Design review of the part shown in the three views and the two pictorial views. Dimensions are in mm from the part's minimum x, y and z. Give positions to 0.01 mm unless a question says otherwise; leave off trailing zeros. Order: outer loops, then holes, each group sorted by start corner. A loop starts at its lowest first (then second) coordinate and runs counter-clockwise, first axis right, second up. Notation, with made-up numbers: (-10, -30.75) - (29, -30.75) arc R29 cw to (29, -10.75) - close; hole circle Ø3 at (11.25, 6). An arc over 180 degrees is marked (long way). Put each result on its own line as item: value.
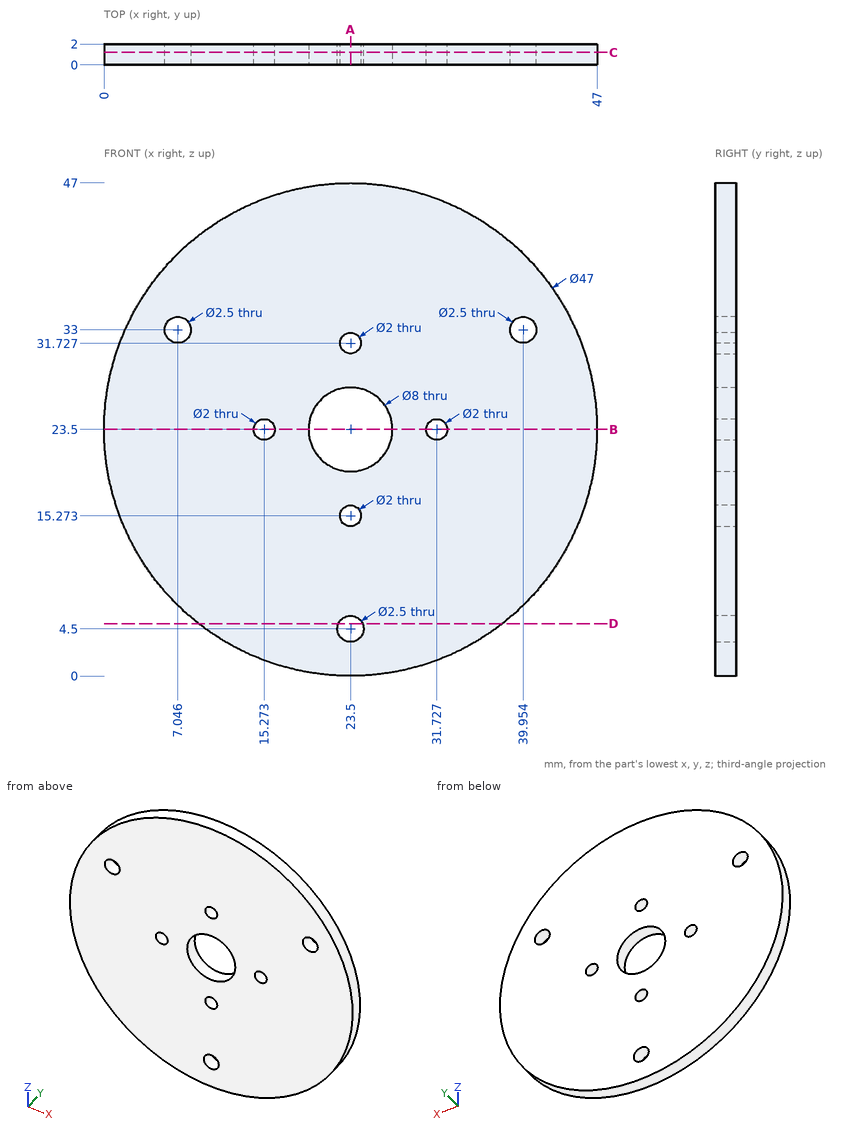
(1) Take a section at D-D, the plane z = 5. Write out the cut boundary in (x, y) (1 decimal).
The answers:
outline: (9, 0) - (22.4, 0) - (22.4, 2) - (9, 2) - close; (24.6, 0) - (38, 0) - (38, 2) - (24.6, 2) - close
(2) Wall thickness on L1, parallel to X at y = 0.95, z = 23.5; L2, parallel to X at y = 1.1, z = 33 (1 decimal); L3, parallel to X at y = 0.75, z = 33.5 (1 decimal): over which ranges is each line inside the solid? List them lowest first.
The answers:
L1: 0 to 14.27, 16.27 to 19.5, 27.5 to 30.73, 32.73 to 47
L2: 2 to 5.8, 8.3 to 38.7, 41.2 to 45
L3: 2.2 to 5.9, 8.2 to 38.8, 41.1 to 44.8
(3) Take a section at A-A, the plane x = 23.5. Write out the cut boundary in (y, z).
The answers:
outline: (0, 0) - (2, 0) - (2, 3.25) - (0, 3.25) - close; (0, 5.75) - (2, 5.75) - (2, 14.27) - (0, 14.27) - close; (0, 16.27) - (2, 16.27) - (2, 19.5) - (0, 19.5) - close; (0, 27.5) - (2, 27.5) - (2, 30.73) - (0, 30.73) - close; (0, 32.73) - (2, 32.73) - (2, 47) - (0, 47) - close
(4) Take a section at C-C, the plane y = 1.2. Count the separate pieces of the cut face and the enclosed holes in it, then the cut area to 3 significant figures.
The answers:
separate pieces: 1
enclosed holes: 8
area: 1,660 mm^2
(5) Take a section at B-B, the plane z = 23.5. Write out the cut boundary in (x, y).
The answers:
outline: (0, 0) - (14.27, 0) - (14.27, 2) - (0, 2) - close; (16.27, 0) - (19.5, 0) - (19.5, 2) - (16.27, 2) - close; (27.5, 0) - (30.73, 0) - (30.73, 2) - (27.5, 2) - close; (32.73, 0) - (47, 0) - (47, 2) - (32.73, 2) - close
